from build123d import *

# Parameters (mm, degrees)
SKETCH_1_W               = 285
SKETCH_1_H               = 70
EXTRUDE_1_DEPTH          = 2.7
SKETCH_2_R               = 1.6
SKETCH_2_R_2             = 7.5
CUT_EXTRUDE_1_DEPTH      = 147.760144453
PATTERN_LINEAR_1_COUNT   = 8
PATTERN_LINEAR_1_PITCH   = 35
SKETCH_5_W               = 4
SKETCH_5_H               = 8
SKETCH_5_W_2             = 8
EXTRUDE_3_DEPTH          = 6
CUT_EXTRUDE_3_DEPTH      = 284.304941715
CUT_EXTRUDE_3_DEPTH_BACK = 284.304941715
SKETCH_7_R               = 1.6
SKETCH_7_R_2             = 1.25
SKETCH_9_R               = 3
EXTRUDE_4_DEPTH          = 2.7
CUT_EXTRUDE_4_DEPTH      = 147.857924539
PATTERN_LINEAR_2_COUNT   = 7
PATTERN_LINEAR_2_PITCH   = 35
PATTERN_LINEAR_3_COUNT   = 2
PATTERN_LINEAR_3_PITCH   = 35
CUT_EXTRUDE_2_DEPTH      = 147.857924539
CUT_EXTRUDE_2_DEPTH_BACK = 147.857924539


with BuildPart() as part:
    # 草图1 → 凸台-拉伸1 (new body)
    with BuildSketch(Plane.XY):
        Rectangle(SKETCH_1_W, SKETCH_1_H)
    extrude(amount=EXTRUDE_1_DEPTH)

    # 草图2 → 切除-拉伸1 (cut, through all)
    with BuildSketch(Plane.XY.offset(2.7)):
        with Locations((-106.5, -32)):
            Circle(SKETCH_2_R)
        with Locations((-106.5, 30)):
            Circle(SKETCH_2_R)
        with Locations((-126.5, 18)):
            Circle(SKETCH_2_R_2)
        with BuildLine():
            Line((-125.560660172, -30.939339828), (-88.560660172, 6.060660172))
            ThreePointArc((-88.560660172, 6.060660172), (-86.439339828, 6.060660172), (-86.439339828, 3.939339828))
            Line((-86.439339828, 3.939339828), (-123.439339828, -33.060660172))
            ThreePointArc((-123.439339828, -33.060660172), (-125.560660172, -33.060660172), (-125.560660172, -30.939339828))
        make_face()
    cut_extrude_1 = extrude(amount=-CUT_EXTRUDE_1_DEPTH, mode=Mode.SUBTRACT)

    # 阵列(线性)1: 切除-拉伸1 ×8
    with Locations(*[(i * PATTERN_LINEAR_1_PITCH, 0, 0) for i in range(1, PATTERN_LINEAR_1_COUNT)]):
        add(cut_extrude_1, mode=Mode.SUBTRACT)

    # 草图5 → 凸台-拉伸3 (add)
    with BuildSketch(Plane.XY.offset(2.7)):
        with Locations((-140.5, -31)):
            Rectangle(SKETCH_5_W, SKETCH_5_H)
        with Locations((140.5, -31)):
            Rectangle(SKETCH_5_W, SKETCH_5_H)
        with Locations((7, -31)):
            Rectangle(SKETCH_5_W_2, SKETCH_5_H)
        with Locations((-140.5, 13)):
            Rectangle(SKETCH_5_W, SKETCH_5_H)
        with Locations((140.5, 13)):
            Rectangle(SKETCH_5_W, SKETCH_5_H)
        with Locations((-4, 13)):
            Rectangle(SKETCH_5_W, SKETCH_5_H)
    extrude(amount=EXTRUDE_3_DEPTH)

    # 草图7 → 切除-拉伸3 (cut, two sides: drawn at the far end of the back side and taken through both)
    with BuildSketch(Plane(origin=(-138.5, 0, 0), x_dir=(0, 0, -1), z_dir=(1, 0, 0)).offset(-CUT_EXTRUDE_3_DEPTH_BACK)):
        with Locations(Location((-5.7, -32, 0), (0, 0, 270))):
            Circle(SKETCH_7_R)
        with Locations(Location((-5.7, 13, 0), (0, 0, 270))):
            Circle(SKETCH_7_R_2)
    extrude(amount=CUT_EXTRUDE_3_DEPTH + CUT_EXTRUDE_3_DEPTH_BACK, mode=Mode.SUBTRACT)

    # 草图9 → 凸台-拉伸4 (add)
    with BuildSketch(Plane.XY.offset(2.7)):
        with Locations((138.5, -32)):
            Circle(SKETCH_9_R)
        with BuildLine():
            Line((137.196699141, -13.181980515), (142.5, -7.878679656))
            Line((142.5, -7.878679656), (142.5, -12.121320344))
            Line((142.5, -12.121320344), (139.318019485, -15.303300859))
            ThreePointArc((139.318019485, -15.303300859), (139.318019485, -13.181980515), (137.196699141, -13.181980515))
        make_face()
    extrude(amount=-EXTRUDE_4_DEPTH)

    # 草图10 → 切除-拉伸4 (cut, through all)
    with BuildSketch(Plane.XY.offset(2.7)):
        with BuildLine():
            Line((-100.121320344, -20.878679656), (-75.372583002, 3.870057685))
            ThreePointArc((-75.372583002, 3.870057685), (-71.129942315, 3.870057685), (-71.129942315, -0.372583002))
            Line((-71.129942315, -0.372583002), (-95.878679656, -25.121320344))
            ThreePointArc((-95.878679656, -25.121320344), (-100.121320344, -25.121320344), (-100.121320344, -20.878679656))
        make_face()
    cut_extrude_4 = extrude(amount=-CUT_EXTRUDE_4_DEPTH, mode=Mode.SUBTRACT)

    # 阵列(线性)2: 切除-拉伸4 ×7, 1 skipped
    with Locations(*[(i * PATTERN_LINEAR_2_PITCH, 0, 0) for i in range(1, PATTERN_LINEAR_2_COUNT) if i not in (3,)]):
        add(cut_extrude_4, mode=Mode.SUBTRACT)

    # 阵列(线性)3: 切除-拉伸4 ×2
    with Locations(*[(-i * PATTERN_LINEAR_3_PITCH, 0, 0) for i in range(1, PATTERN_LINEAR_3_COUNT)]):
        add(cut_extrude_4, mode=Mode.SUBTRACT)

    # 草图3 → 切除-拉伸2 (cut, two sides: drawn at the far end of the back side and taken through both)
    with BuildSketch(Plane.XY.offset(2.7).offset(-CUT_EXTRUDE_2_DEPTH_BACK)):
        Polygon((27.5, 35), (-142.5, 35), (-142.5, -35), (7, -35), (7, -23), (27.5, -2.5), align=None)
    extrude(amount=CUT_EXTRUDE_2_DEPTH + CUT_EXTRUDE_2_DEPTH_BACK, mode=Mode.SUBTRACT)


solid = part.part
Design review of the part built by this model. Coordinates are the model's own, in mm. A direction names the side the tool comes from. Coordinates: 2 decimals unless noted, no trailing zeros. Order: outer loops, then holes, each group sorted by start corner. A loop starts at its lowest first (then second) coordinate and runs counter-clockwise, first axis right, second up.
Item 1: Take a section at C-C, the plane x = 131. Write out the cut boundary in (y, z).
Item 2: The part is to be moulded in two halves that separate along X. For faces 4 (the cylindrical face through (70.026, 30.481, 1.369)), 5 (the flat face through (140, 13, 8.7)), say which applies: pulls with the +X half, pulls with the -X half, needs draft (parallel to the pull), parting line crosses it, or undercut.
Item 3: Take a section at B-B, the plane x = 33.5. Write out the cut boundary in (y, z), then the cut area to 3 significant figures.
Item 4: For line 1 (Y direction, x = 118.5, z = 2.15); line 2 (Y direction, x = 68.5, z = 1.35); line 3 (Y direction, x = 33.5, z = 0.9), list the stretches that pass through material, from the lowest coordinate up.
Item 5: For pin 1 Ø2.5 at (y, z) = (-32, 5.7) entering from -X; pin 2 Ø1.2 at (x, z) = (9.5, 7) entering from +Y; pin 3 Ø3 at (y, z) = (12.5, 7) entering from -X; pin 4 Ø2 at (y, z) = (20, 1.5) entering from -X, all flat-tipped, find the tip position at first contact; note any pin that passes through.
Item 6: Take a section at A-A, the plane y = 30. Write out the cut boundary in (x, z).
Item 7: Take a section at D-D, the plane x = 18.5. Write out the cut boundary in (y, z), then the cut area to 3 significant figures.
Item 8: For faces 1 (the flat face through (140, 17, 6)), 2 (the flat face through (130.56, -24.06, 1.37)), 3 (the flat face through (138.5, -30, 6)), list the 3-axis set-ups (+Z, -Z, +X, -X, +Y, -Y) from which the entire face can be reached by the end or side of a thin tool; tool diameter is ignored.
The answers:
1. outline: (-35, 0) - (-23.62, 0) - (-23.62, 2.7) - (-35, 2.7) - close; (-19.38, 0) - (-8.24, 0) - (-8.24, 2.7) - (-19.38, 2.7) - close; (0.24, 0) - (35, 0) - (35, 2.7) - (0.24, 2.7) - close
2. face 4: undercut
2. face 5: needs draft
3. outline: (-35, 0) - (-33.6, 0) - (-33.6, 2.7) - (-35, 2.7) - close; (-30.4, 0) - (-16.12, 0) - (-16.12, 2.7) - (-30.4, 2.7) - close; (-11.88, 0) - (28.4, 0) - (28.4, 2.7) - (-11.88, 2.7) - close; (31.6, 0) - (35, 0) - (35, 2.7) - (31.6, 2.7) - close
3. area: 160 mm2
4. line 1: y = -35 to -20.74, -12.26 to -1.12, 3.12 to 10.5, 25.5 to 35
4. line 2: y = -35 to -33.6, -30.4 to -16.12, -11.88 to -0.74, 4.18 to 28.4, 31.6 to 35
4. line 3: y = -35 to -33.6, -30.4 to -16.12, -11.88 to 28.4, 31.6 to 35
5. pin 1: passes through
5. pin 2: stops at y = -27
5. pin 3: stops at x = 138.5
5. pin 4: stops at x = 27.5
6. outline: (27.5, 0) - (31.9, 0) - (31.9, 2.7) - (27.5, 2.7) - close; (35.1, 0) - (66.9, 0) - (66.9, 2.7) - (35.1, 2.7) - close; (70.1, 0) - (101.9, 0) - (101.9, 2.7) - (70.1, 2.7) - close; (105.1, 0) - (136.9, 0) - (136.9, 2.7) - (105.1, 2.7) - close; (140.1, 0) - (142.5, 0) - (142.5, 2.7) - (140.1, 2.7) - close
7. outline: (-35, 0) - (-31.12, 0) - (-31.12, 2.7) - (-35, 2.7) - close; (-26.88, 0) - (-11.5, 0) - (-11.5, 2.7) - (-26.88, 2.7) - close
7. area: 52.0 mm2
8. face 1: +Z, +X, -X, +Y
8. face 2: +Z, -Z
8. face 3: +Z, +Y, -Y
